from build123d import *

# Parameters (mm, degrees)
EXTRUDE_1_DEPTH     = 5
SKETCH_2_R          = 1.6
CUT_EXTRUDE_2_DEPTH = 205.826540078
FILLET_1_R          = 5


with BuildPart() as part:
    # 草圖1 → 伸長1 (new body)
    with BuildSketch(Plane(origin=(0, 0, 0), x_dir=(1, 0, 0), z_dir=(0, 1, 0))):
        with BuildLine():
            Line((0, 50), (0, 100))
            ThreePointArc((0, 100), (24.455049934, 158.55833165), (83.293389788, 182.331792401))
            ThreePointArc((83.293389788, 182.331792401), (93.176602271, 172.216353161), (83.061163031, 162.333140678))
            ThreePointArc((83.061163031, 162.333140678), (38.514841271, 144.334328431), (20, 100))
            Line((20, 100), (20, 50))
            Line((20, 50), (20, 0))
            Line((20, 0), (0, 0))
            Line((0, 0), (0, 50))
        make_face()
    extrude(amount=EXTRUDE_1_DEPTH)

    # 草圖2 → 伸長2 (cut, through all)
    with BuildSketch(Plane(origin=(0, 5, 0), x_dir=(1, 0, 0), z_dir=(0, 1, 0))):
        with Locations(Location((10, 60, 0), (0, 0, 270))):
            Circle(SKETCH_2_R)
        with Locations(Location((10, 30, 0), (0, 0, 270))):
            Circle(SKETCH_2_R)
        with Locations(Location((83.177276409, 172.33246654, 0), (0, 0, 270))):
            Circle(SKETCH_2_R)
        with Locations(Location((10, 100, 0), (0, 0, 270))):
            Circle(SKETCH_2_R)
    extrude(amount=-CUT_EXTRUDE_2_DEPTH, mode=Mode.SUBTRACT)

    # 圓角1
    fillet_1_edges = [part.edges().sort_by_distance(p)[0] for p in [
        (20, 2.5, 0),
        (0, 2.5, 0),
    ]]
    fillet(fillet_1_edges, radius=FILLET_1_R)


solid = part.part
Could you check a few things on this model? Use its own coordinates, in mm. Give positions to 0.01 mm unless a question says otherwise; leave off trailing zeros. Write each loop counter-clockwise with the first axis right and the second up, starting at its lowest first coordinate (ties: lowest second). Pieces come first, ordered by that corner, then holes. Notation, with made-up numbers: (72, -12.5) -> (106, -12.5) arc R20 cw to (106, -2.5) -> close; hole circle Ø7 at (47, 18). An arc over 180 degrees is marked (long way). Write each question's results on one line, items separated by ' | '. Start each with the question number.
Q1. I'm going to push flat-ended pins straight in: pin 1 Ø2 at (y, z) = (1.5, -56) entering from +X; pin 2 Ø2.5 at (x, z) = (83.18, -172.33) entering from +Y; pin 3 Ø2 at (x, y) = (24.5, 4) entering from -Z. Where does each tip first touch, or does it pass through?
Q2. Suppose I cut it at B-B, the plane z = -92. List the corners of the cut face in (x, y) for me, and give its area (3 significant figures).
Q3. I need wall thicknesses on probe 1 along X at (y, z) = (1.7, -100); probe 2 along Z at (x, y) = (9.5, 0.3); probe 3 along X at (y, z) = (0.85, -38). Which ranges of each line are inside material? Lowest first, please.
Q4. We'd pull the mould along X, two halves only. Please class faces 1 (the face through (19, 0, -98)), 2 (the face through (9.39, 2.54, -58.52)), 3 (the face through (0, 2, -52)), 4 (the face through (20, 2, -53)): +X half, -X half, draft (parallel to the pull), parting line (faces both ways), or undercut.
Q5. Suppose I cut it at A-A, the plane y = 2.15. List the corners of the cut face in (x, z) for me, and give its area (3 significant figures).
Q6. Suppose I cut it at C-C, the plane x = 25. List the corners of the cut face in (y, z) for me.
Outcome:
1) pin 1: x = 20 | pin 2: through | pin 3: z = -159.57
2) outline: (0, 0) -> (20, 0) -> (20, 5) -> (0, 5) -> close | area: 100 mm2
3) probe 1: 0 to 8.4, 11.6 to 20 | probe 2: -138.39 to -101.52, -98.48 to -61.52, -58.48 to -31.52, -28.48 to 0 | probe 3: 0 to 20
4) face 1: draft | face 2: undercut | face 3: -X half | face 4: +X half
5) outline: (0, -100) arc R82.34 ccw to (83.29, -182.33) arc R10 ccw to (83.06, -162.33) arc R62.34 cw to (20, -100) -> (20, -5) arc R5 ccw to (15, 0) -> (5, 0) arc R5 ccw to (0, -5) -> close; hole circle Ø3.2 at (10, -100); hole circle Ø3.2 at (10, -60); hole circle Ø3.2 at (10, -30); hole circle Ø3.2 at (83.18, -172.33) | area: 4,400 mm2
6) outline: (0, -159.09) -> (5, -159.09) -> (5, -124.46) -> (0, -124.46) -> close
